Source: CAD feature listing. Evaluate the final solid. Frame: model axes, mm. Coordinates: 2 decimals unless noted, no trailing zeros. Loops run counter-clockwise (first coordinate to the right, second up) from the corner with the lowest first, then second, coordinate; pieces in that order, holes last.
Item 1: Section query D-D, the plane y = 18. Return the cut outline in (x, z).
Item 2: Section query B-B, the plane x = 0. Return the cut outline in (y, z), then the cut area to 3 significant figures.
Item 3: Pin query (flat end, axial travel): pin 1 Ø7 at (y, z) = (66.5, 58.5) entering from -X (3 decimals); pin 2 Ø3 at (x, z) = (-1, 46.5) entering from -Y; pin 3 Ø5 at (x, z) = (-66, 2) entering from -Y. Return the tip coordinate at first contact, or that it passes through.
Item 4: Line query: probe 1 along Y at (x, z) = (0, 3.5); probe 2 along Z at (x, y) = (-43, -46.5); probe 3 along Y at (x, z) = (58.5, 38). Output: solid intervals per line, ascending.
Item 5: Section query A-A, the plane z = 36. Return the cut outline in (x, y) (3 decimals), then the cut area to 3 significant figures.
Item 6: Section query C-C, the plane y = -6. Return the cut outline in (x, z), then the cut area to 3 significant figures.
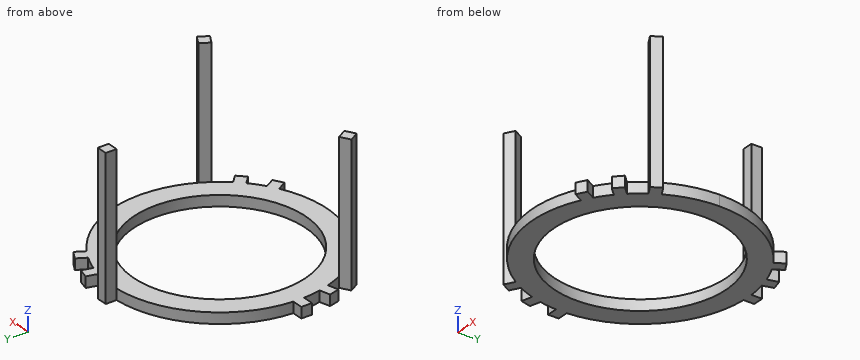
```python
from build123d import *

# Parameters (mm, degrees)
F0_R     = 50.8
F1_DEPTH = 6.35
F2_W     = 6.35
F2_H     = 6.4294246715
F3_DEPTH = 76.2


# Not quite as in the source:
# - a feature names something its author has since deleted; it is built from what else it names


with BuildPart() as f1:
    # F0 (on Top) → F1 (new body)
    with BuildSketch(Plane.XY):
        with BuildLine():
            ThreePointArc((56.5113293571, -28.9606570072), (61.7281111576, -14.895982442), (63.5, 0))
            ThreePointArc((63.5, 0), (55.7694128237, 30.3648249344), (34.4599183213, 53.3363293571))
            Line((34.4599183213, 53.3363293571), (31.324630657, 47.9058518263))
            Line((31.324630657, 47.9058518263), (25.825369343, 51.0808518263))
            Line((25.825369343, 51.0808518263), (28.9606570072, 56.5113293571))
            ThreePointArc((28.9606570072, 56.5113293571), (24.3003979552, 58.6663503145), (19.4812672448, 60.4378211597))
            Line((19.4812672448, 60.4378211597), (17.8583229261, 54.3809105042))
            Line((17.8583229261, 54.3809105042), (11.7246939291, 56.0244114406))
            Line((11.7246939291, 56.0244114406), (13.3476382479, 62.0813220961))
            ThreePointArc((13.3476382479, 62.0813220961), (8.288413206, 62.9567486972), (3.175, 63.4205753285))
            Line((3.175, 63.4205753285), (3.175, 57.15))
            Line((3.175, 57.15), (-3.175, 57.15))
            Line((-3.175, 57.15), (-3.175, 63.4205753285))
            ThreePointArc((-3.175, 63.4205753285), (-44.9012806053, 44.9012806053), (-63.4205753285, 3.175))
            Line((-63.4205753285, 3.175), (-57.15, 3.175))
            Line((-57.15, 3.175), (-57.15, -3.175))
            Line((-57.15, -3.175), (-63.4205753285, -3.175))
            ThreePointArc((-63.4205753285, -3.175), (-62.9567486972, -8.288413206), (-62.0813220961, -13.3476382479))
            Line((-62.0813220961, -13.3476382479), (-56.0244114406, -11.7246939291))
            Line((-56.0244114406, -11.7246939291), (-54.3809105042, -17.8583229261))
            Line((-54.3809105042, -17.8583229261), (-60.4378211597, -19.4812672448))
            ThreePointArc((-60.4378211597, -19.4812672448), (-58.6663503145, -24.3003979552), (-56.5113293571, -28.9606570072))
            Line((-56.5113293571, -28.9606570072), (-51.0808518263, -25.825369343))
            Line((-51.0808518263, -25.825369343), (-47.9058518263, -31.324630657))
            Line((-47.9058518263, -31.324630657), (-53.3363293571, -34.4599183213))
            ThreePointArc((-53.3363293571, -34.4599183213), (-16.435009364, -61.3362899694), (28.9606570072, -56.5113293571))
            Line((28.9606570072, -56.5113293571), (25.825369343, -51.0808518263))
            Line((25.825369343, -51.0808518263), (31.324630657, -47.9058518263))
            Line((31.324630657, -47.9058518263), (34.4599183213, -53.3363293571))
            ThreePointArc((34.4599183213, -53.3363293571), (38.6563507421, -50.3779371085), (42.6000548513, -47.0901829118))
            Line((42.6000548513, -47.0901829118), (38.1660885145, -42.6562165751))
            Line((38.1660885145, -42.6562165751), (42.6562165751, -38.1660885145))
            Line((42.6562165751, -38.1660885145), (47.0901829118, -42.6000548513))
            ThreePointArc((47.0901829118, -42.6000548513), (50.3779371085, -38.6563507421), (53.3363293571, -34.4599183213))
            Line((53.3363293571, -34.4599183213), (47.9058518263, -31.324630657))
            Line((47.9058518263, -31.324630657), (51.0808518263, -25.825369343))
            Line((51.0808518263, -25.825369343), (56.5113293571, -28.9606570072))
        make_face()
        Circle(F0_R, mode=Mode.SUBTRACT)
        with BuildLine():
            ThreePointArc((-3.175, 63.4205753285), (0, 63.5), (3.175, 63.4205753285))
            Line((3.175, 63.4205753285), (3.175, 69.85))
            Line((3.175, 69.85), (-3.175, 69.85))
            Line((-3.175, 69.85), (-3.175, 63.4205753285))
        make_face()
        with BuildLine():
            Line((3.175, 57.15), (3.175, 63.4205753285))
            ThreePointArc((3.175, 63.4205753285), (0, 63.5), (-3.175, 63.4205753285))
            Line((-3.175, 63.4205753285), (-3.175, 57.15))
            Line((-3.175, 57.15), (3.175, 57.15))
        make_face()
        with BuildLine():
            Line((17.8583229261, 54.3809105042), (19.4812672448, 60.4378211597))
            ThreePointArc((19.4812672448, 60.4378211597), (16.435009364, 61.3362899694), (13.3476382479, 62.0813220961))
            Line((13.3476382479, 62.0813220961), (11.7246939291, 56.0244114406))
            Line((11.7246939291, 56.0244114406), (17.8583229261, 54.3809105042))
        make_face()
        with BuildLine():
            ThreePointArc((13.3476382479, 62.0813220961), (16.435009364, 61.3362899694), (19.4812672448, 60.4378211597))
            Line((19.4812672448, 60.4378211597), (21.1453247989, 66.6481684981))
            Line((21.1453247989, 66.6481684981), (15.0116958019, 68.2916694345))
            Line((15.0116958019, 68.2916694345), (13.3476382479, 62.0813220961))
        make_face()
        with BuildLine():
            ThreePointArc((28.9606570072, 56.5113293571), (31.75, 54.9926131403), (34.4599183213, 53.3363293571))
            Line((34.4599183213, 53.3363293571), (37.674630657, 58.9043744543))
            Line((37.674630657, 58.9043744543), (32.175369343, 62.0793744543))
            Line((32.175369343, 62.0793744543), (28.9606570072, 56.5113293571))
        make_face()
        with BuildLine():
            Line((31.324630657, 47.9058518263), (34.4599183213, 53.3363293571))
            ThreePointArc((34.4599183213, 53.3363293571), (31.75, 54.9926131403), (28.9606570072, 56.5113293571))
            Line((28.9606570072, 56.5113293571), (25.825369343, 51.0808518263))
            Line((25.825369343, 51.0808518263), (31.324630657, 47.9058518263))
        make_face()
        with BuildLine():
            Line((62.0793744543, -32.175369343), (56.5113293571, -28.9606570072))
            ThreePointArc((56.5113293571, -28.9606570072), (54.9926131403, -31.75), (53.3363293571, -34.4599183213))
            Line((53.3363293571, -34.4599183213), (58.9043744543, -37.674630657))
            Line((58.9043744543, -37.674630657), (62.0793744543, -32.175369343))
        make_face()
        with BuildLine():
            ThreePointArc((53.3363293571, -34.4599183213), (54.9926131403, -31.75), (56.5113293571, -28.9606570072))
            Line((56.5113293571, -28.9606570072), (51.0808518263, -25.825369343))
            Line((51.0808518263, -25.825369343), (47.9058518263, -31.324630657))
            Line((47.9058518263, -31.324630657), (53.3363293571, -34.4599183213))
        make_face()
        with BuildLine():
            Line((51.6364726961, -47.1463446356), (47.0901829118, -42.6000548513))
            ThreePointArc((47.0901829118, -42.6000548513), (44.9012806053, -44.9012806053), (42.6000548513, -47.0901829118))
            Line((42.6000548513, -47.0901829118), (47.1463446356, -51.6364726961))
            Line((47.1463446356, -51.6364726961), (51.6364726961, -47.1463446356))
        make_face()
        with BuildLine():
            ThreePointArc((42.6000548513, -47.0901829118), (44.9012806053, -44.9012806053), (47.0901829118, -42.6000548513))
            Line((47.0901829118, -42.6000548513), (42.6562165751, -38.1660885145))
            Line((42.6562165751, -38.1660885145), (38.1660885145, -42.6562165751))
            Line((38.1660885145, -42.6562165751), (42.6000548513, -47.0901829118))
        make_face()
        with BuildLine():
            ThreePointArc((28.9606570072, -56.5113293571), (31.75, -54.9926131403), (34.4599183213, -53.3363293571))
            Line((34.4599183213, -53.3363293571), (31.324630657, -47.9058518263))
            Line((31.324630657, -47.9058518263), (25.825369343, -51.0808518263))
            Line((25.825369343, -51.0808518263), (28.9606570072, -56.5113293571))
        make_face()
        with BuildLine():
            Line((37.674630657, -58.9043744543), (34.4599183213, -53.3363293571))
            ThreePointArc((34.4599183213, -53.3363293571), (31.75, -54.9926131403), (28.9606570072, -56.5113293571))
            Line((28.9606570072, -56.5113293571), (32.175369343, -62.0793744543))
            Line((32.175369343, -62.0793744543), (37.674630657, -58.9043744543))
        make_face()
        with BuildLine():
            Line((-58.9043744543, -37.674630657), (-53.3363293571, -34.4599183213))
            ThreePointArc((-53.3363293571, -34.4599183213), (-54.9926131403, -31.75), (-56.5113293571, -28.9606570072))
            Line((-56.5113293571, -28.9606570072), (-62.0793744543, -32.175369343))
            Line((-62.0793744543, -32.175369343), (-58.9043744543, -37.674630657))
        make_face()
        with BuildLine():
            ThreePointArc((-60.4378211597, -19.4812672448), (-61.3362899694, -16.435009364), (-62.0813220961, -13.3476382479))
            Line((-62.0813220961, -13.3476382479), (-68.2916694345, -15.0116958019))
            Line((-68.2916694345, -15.0116958019), (-66.6481684981, -21.1453247989))
            Line((-66.6481684981, -21.1453247989), (-60.4378211597, -19.4812672448))
        make_face()
        with BuildLine():
            ThreePointArc((-63.4205753285, -3.175), (-63.5, 0), (-63.4205753285, 3.175))
            Line((-63.4205753285, 3.175), (-69.85, 3.175))
            Line((-69.85, 3.175), (-69.85, -3.175))
            Line((-69.85, -3.175), (-63.4205753285, -3.175))
        make_face()
        with BuildLine():
            Line((-57.15, 3.175), (-63.4205753285, 3.175))
            ThreePointArc((-63.4205753285, 3.175), (-63.5, 0), (-63.4205753285, -3.175))
            Line((-63.4205753285, -3.175), (-57.15, -3.175))
            Line((-57.15, -3.175), (-57.15, 3.175))
        make_face()
        with BuildLine():
            Line((-56.0244114406, -11.7246939291), (-62.0813220961, -13.3476382479))
            ThreePointArc((-62.0813220961, -13.3476382479), (-61.3362899694, -16.435009364), (-60.4378211597, -19.4812672448))
            Line((-60.4378211597, -19.4812672448), (-54.3809105042, -17.8583229261))
            Line((-54.3809105042, -17.8583229261), (-56.0244114406, -11.7246939291))
        make_face()
        with BuildLine():
            ThreePointArc((-56.5113293571, -28.9606570072), (-54.9926131403, -31.75), (-53.3363293571, -34.4599183213))
            Line((-53.3363293571, -34.4599183213), (-47.9058518263, -31.324630657))
            Line((-47.9058518263, -31.324630657), (-51.0808518263, -25.825369343))
            Line((-51.0808518263, -25.825369343), (-56.5113293571, -28.9606570072))
        make_face()
    extrude(amount=F1_DEPTH)

    # F2 (on face) → F3 (join)
    with BuildSketch(Plane.XY.offset(6.35)):
        with Locations((0, 66.6352876643)):
            Rectangle(F2_W, F2_H)
        Polygon((62.0793744543, -32.175369343), (56.5113293571, -28.9606570072), (53.3363293571, -34.4599183213), (58.9043744543, -37.674630657), align=None)
        Polygon((-53.3363293571, -34.4599183213), (-56.5113293571, -28.9606570072), (-62.0793744543, -32.175369343), (-58.9043744543, -37.674630657), align=None)
    extrude(amount=F3_DEPTH)


solid = f1.part
```
Verdict:
1. outline: (-60.9, 0) - (-47.5, 0) - (-47.5, 6.35) - (-60.9, 6.35) - close; (47.5, 0) - (60.9, 0) - (60.9, 6.35) - (47.5, 6.35) - close
2. outline: (-63.5, 0) - (-50.8, 0) - (-50.8, 6.35) - (-63.5, 6.35) - close; (50.8, 0) - (69.85, 0) - (69.85, 82.55) - (63.42, 82.55) - (63.42, 6.35) - (50.8, 6.35) - close
2. area: 692 mm2
3. pin 1: stops at x = -3.175
3. pin 2: stops at y = 63.42
3. pin 3: stops at y = -21.15
4. probe 1: y = -63.5 to -50.8, 50.8 to 69.85
4. probe 2: z = 0 to 6.35
4. probe 3: y = -37.44 to -30.11
5. outline: (-62.079, -32.175) - (-58.904, -37.675) - (-53.336, -34.46) - (-56.511, -28.961) - close; (-3.175, 63.421) - (3.175, 63.421) - (3.175, 69.85) - (-3.175, 69.85) - close; (53.336, -34.46) - (58.904, -37.675) - (62.079, -32.175) - (56.511, -28.961) - close
5. area: 122 mm2
6. outline: (-63.22, 0) - (-50.44, 0) - (-50.44, 6.35) - (-63.22, 6.35) - close; (50.44, 0) - (63.22, 0) - (63.22, 6.35) - (50.44, 6.35) - close
6. area: 162 mm2
